Source: CAD feature listing. Evaluate the final solid. Frame: model axes, mm. A direction names the side the tool comes from. Give positions to 0.01 mm unless a question says otherwise; leave off trailing zeros. Loops run counter-clockwise (first coordinate to the right, second up) from the corner with the lowest first, then second, coordinate; pieces in that order, holes last. Notation, with made-up numbers: (11, 30.5) -> (50, 30.5) arc R26 ccw to (50, 46.5) -> close; hole circle Ø11 at (38.5, 68.5). An arc over 180 degrees is marked (long way). Put each result on its own line as item: value.
```python
from build123d import *

# Parameters (mm, degrees)
SKETCH1_R               = 9.5
SKETCH1_R_2             = 8.25
BOSS_EXTRUDE1_DEPTH     = 4
SKETCH2_R               = 11.25
BOSS_EXTRUDE2_DEPTH     = 2
CUT_EXTRUDE1_DEPTH      = 18.003676073
CUT_EXTRUDE1_DEPTH_BACK = 18.003676073
SKETCH3_R               = 5.4
CHAMFER1_SIZE           = 1.5
CHAMFER2_SIZE           = 0.5
CHAMFER3_SIZE           = 1


with BuildPart() as part:
    # Sketch1 → Boss-Extrude1 (new body)
    with BuildSketch(Plane(origin=(0, 0, 0), x_dir=(1, 0, 0), z_dir=(0, 1, 0))):
        with Locations(Location((0, 0, 0), (0, 0, 270))):
            Circle(SKETCH1_R)
        with Locations(Location((0, 0, 0), (0, 0, 270))):
            Circle(SKETCH1_R_2, mode=Mode.SUBTRACT)
    extrude(amount=BOSS_EXTRUDE1_DEPTH)

    # Sketch2 → Boss-Extrude2 (add)
    with BuildSketch(Plane(origin=(0, 4, 0), x_dir=(1, 0, 0), z_dir=(0, 1, 0))):
        with Locations(Location((0, 0, 0), (0, 0, 270))):
            Circle(SKETCH2_R)
    extrude(amount=BOSS_EXTRUDE2_DEPTH)

    # Sketch3 → Cut-Extrude1 (cut, two sides: drawn at the far end of the back side and taken through both)
    with BuildSketch(Plane(origin=(0, 6, 0), x_dir=(1, 0, 0), z_dir=(0, 1, 0)).offset(-CUT_EXTRUDE1_DEPTH_BACK)):
        with Locations(Location((0, 0, 0), (0, 0, 270))):
            Circle(SKETCH3_R)
    extrude(amount=CUT_EXTRUDE1_DEPTH + CUT_EXTRUDE1_DEPTH_BACK, mode=Mode.SUBTRACT)

    # Chamfer1
    chamfer1_edges = [part.edges().sort_by_distance(p)[0] for p in [
        (0, 4, -5.4),
    ]]
    chamfer(chamfer1_edges, length=CHAMFER1_SIZE)

    # Chamfer2
    chamfer2_edges = [part.edges().sort_by_distance(p)[0] for p in [
        (0, 0, -9.5),
        (0, 0, -8.25),
    ]]
    chamfer(chamfer2_edges, length=CHAMFER2_SIZE)

    # Chamfer3
    # the kernel refuses this chamfer: 1 mm, written as the material it takes off along each edge
    with BuildSketch(Plane(origin=(0, 6, 0), x_dir=(0, 0, 1), z_dir=(-1, 0, 0))) as chamfer3_piece_1:
        Polygon((11.25 - CHAMFER3_SIZE, 0), (11.25, -CHAMFER3_SIZE), (11.25, 0), align=None)
    revolve(axis=Axis((0, 6, 0), (0, 1, 0)), mode=Mode.SUBTRACT)
    with BuildSketch(Plane(origin=(0, 6, 0), x_dir=(0, 0, 1), z_dir=(-1, 0, 0))) as chamfer3_piece_2:
        Polygon((5.4, -CHAMFER3_SIZE), (5.4 + CHAMFER3_SIZE, 0), (5.4, 0), align=None)
    revolve(axis=Axis((0, 6, 0), (0, 1, 0)), mode=Mode.SUBTRACT)


solid = part.part
```
(1) Section C-C on y = 2.4. Return loops of the section in (x, z), then the cut area to 3 significant figures.
Calculated:
outline: circle Ø19 at (0, 0); hole circle Ø16.5 at (0, 0)
area: 69.7 mm²
(2) Section A-A on x = 0. Return loops of the section in (y, z), then the cut area to 3 significant figures.
Calculated:
outline: (0, -9) -> (0.5, -9.5) -> (4, -9.5) -> (4, -11.25) -> (5, -11.25) -> (6, -10.25) -> (6, -6.4) -> (5.25, -5.65) -> (4, -6.9) -> (4, -8.25) -> (0.5, -8.25) -> (0, -8.75) -> close; (0, 8.75) -> (0.5, 8.25) -> (4, 8.25) -> (4, 6.9) -> (5.25, 5.65) -> (6, 6.4) -> (6, 10.25) -> (5, 11.25) -> (4, 11.25) -> (4, 9.5) -> (0.5, 9.5) -> (0, 9) -> close
area: 28.8 mm²
(3) Section B-B on z = 0. Return loops of the section in (x, y), then the cut area to 3 significant figures.
Calculated:
outline: (-11.25, 4) -> (-9.5, 4) -> (-9.5, 0.5) -> (-9, 0) -> (-8.75, 0) -> (-8.25, 0.5) -> (-8.25, 4) -> (-6.9, 4) -> (-5.65, 5.25) -> (-6.4, 6) -> (-10.25, 6) -> (-11.25, 5) -> close; (5.65, 5.25) -> (6.9, 4) -> (8.25, 4) -> (8.25, 0.5) -> (8.75, 0) -> (9, 0) -> (9.5, 0.5) -> (9.5, 4) -> (11.25, 4) -> (11.25, 5) -> (10.25, 6) -> (6.4, 6) -> close
area: 28.8 mm²
(4) Line query: probe 1 along X at (y, z) = (3.2, 0); probe 2 along X at (y, z) = (2.9, 4.25); probe 3 along Z at (x, y) = (-1, 0.55). Output: solid intervals per line, ascending. Write a range as from..to.
Calculated:
probe 1: x = -9.5..-8.25, 8.25..9.5
probe 2: x = -8.5..-7.07, 7.07..8.5
probe 3: z = -9.45..-8.19, 8.19..9.45
(5) Draft query along Z for faces 1 (the flat face through (-6, 4, -8)), 2 (the cylindrical face through (-8.054, 2.226, -1.788)), 3 (the cylindrical face through (-4.31, 4.49, 10.39)). Return one class per face: released by +Z, released by -Z, zero draft, split by the parting line, or undercut.
Calculated:
face 1: zero draft
face 2: undercut
face 3: split by the parting line
(6) First-contact query: P1, Ø6, axis at x = -4, z = -7.5, coming from the -Y side; P2, Ø5, axis at x = -2.5, z = -0.5, coming from the -Y side. Flat tips, straight axial feed; report the tip coordinate or a pass-through.
Calculated:
P1: stops at y = 0
P2: passes through
(7) Reachability of faces 4 (the flat face through (0, 6, 7)), 5 (the flat face through (-7, 4, -2)) from +Z, -Z, +X, -X, +Y, -Y: full face, straight path, thin tool, end or side. Return the list, or none.
Calculated:
face 4: +Z, -Z, +X, -X, +Y
face 5: -Y
